Geometry: final body of the model. Coordinates: model frame, mm. Give positions to 0.01 mm unless a question says otherwise; leave off trailing zeros. Loops run counter-clockwise (first coordinate to the right, second up) from the corner with the lowest first, then second, coordinate; pieces in that order, holes last. Notation, with made-up numbers: M 57,-19 L 85,-19 A22 ccw 85,-7 Z; hole C 40.5,-17.75 d9. An arc over 180 degrees is marked long. Put each result on its own line as item: value.
```python
from build123d import *

# Parameters (mm, degrees)
BOSS_EXTRUDE1_DEPTH = 20
SKETCH7_R           = 15
CUT_EXTRUDE1_DEPTH  = 20
SKETCH6_R           = 3
CUT_EXTRUDE2_DEPTH  = 24


with BuildPart() as part:
    # Sketch1 → Boss-Extrude1 (new body)
    with BuildSketch(Plane(origin=(0, 0, 0), x_dir=(0, 0, -1), z_dir=(1, 0, 0))):
        Polygon((0, 0), (-30, 0), (-30, 24), (30, 24), (30, 0), align=None)
    extrude(amount=-BOSS_EXTRUDE1_DEPTH)

    # Sketch7 → Cut-Extrude1 (cut)
    with BuildSketch(Plane.ZY.offset(20)):
        Circle(SKETCH7_R)
    extrude(amount=-CUT_EXTRUDE1_DEPTH, mode=Mode.SUBTRACT)

    # Sketch6 → Cut-Extrude2 (cut)
    with BuildSketch(Plane(origin=(0, 24, 0), x_dir=(1, 0, 0), z_dir=(0, 1, 0))):
        with Locations(Location((-10.527062393, 26, 0), (0, 0, 270))):
            Circle(SKETCH6_R)
        with Locations(Location((-10.527062393, -26, 0), (0, 0, 270))):
            Circle(SKETCH6_R)
    extrude(amount=-CUT_EXTRUDE2_DEPTH, mode=Mode.SUBTRACT)


solid = part.part
```
Item 1: Section C-C on x = -15.5. Output: boundary loops of the cut face in (y, z), then the cut area to 3 significant figures.
Output values:
outline: M 0,-30 L 24,-30 L 24,30 L 0,30 L 0,15 A15 cw 0,-15 Z
area: 1,090 mm²
Item 2: Mould query, pull axis Z, two halves, no side actions, for faces 1 (the cylindrical face through (-10, 15, 0)), 2 (the cylindrical face through (-12.353, 12.168, -28.381)), 3 (the flat face through (-10, 12, 30)), 4 (the flat face through (0, 18, 0)). Classes: pulls with the +Z half, pulls with the -Z half, needs draft (parallel to the pull), parting line crosses it, or undercut.
Output values:
face 1: undercut
face 2: undercut
face 3: pulls with the +Z half
face 4: needs draft
Item 3: Section B-B on y = 8.25. Output: boundary loops of the cut face in (x, z).
Output values:
outline: M -20,-30 L 0,-30 L 0,-12.53 L -20,-12.53 Z; M -20,12.53 L 0,12.53 L 0,30 L -20,30 Z; hole C -10.53,-26 d6; hole C -10.53,26 d6
Item 4: Line query: probe 1 along X at (y, z) = (5, -26); probe 2 along Z at (x, y) = (-10.75, 2.5); probe 3 along Z at (x, y) = (-8.75, 20.75). Output: solid intervals per line, ascending. Write a range as [from, to].
Output values:
probe 1: [-20, -13.53], [-7.53, 0]
probe 2: [-30, -28.99], [-23.01, -14.79], [14.79, 23.01], [28.99, 30]
probe 3: [-30, -28.42], [-23.58, 23.58], [28.42, 30]
Item 5: Section D-D on y = 13.5. Output: boundary loops of the cut face in (x, z).
Output values:
outline: M -20,-30 L 0,-30 L 0,-6.54 L -20,-6.54 Z; M -20,6.54 L 0,6.54 L 0,30 L -20,30 Z; hole C -10.53,-26 d6; hole C -10.53,26 d6
Item 6: Section A-A on z = -26. Output: boundary loops of the cut face in (x, y), then the cut area to 3 significant figures.
Output values:
outline: M -20,0 L -13.53,0 L -13.53,24 L -20,24 Z; M -7.53,0 L 0,0 L 0,24 L -7.53,24 Z
area: 336 mm²
Item 7: Pin query (flat end, axial travel): pin 1 Ø8 at (x, z) = (-9.5, -5) entering from -Y; pin 2 Ø8 at (y, z) = (3, 11.5) entering from +X; pin 3 Ø3.5 at (x, z) = (-10.53, 26) entering from +Y; pin 4 Ø3 at (x, z) = (-17.5, 11) entering from -Y. Return the tip coordinate at first contact, or that it passes through.
Output values:
pin 1: y = 12
pin 2: x = 0
pin 3: through
pin 4: y = 8.29
